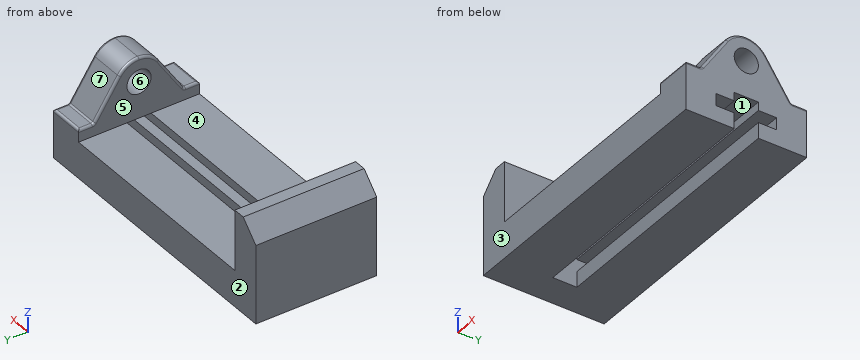
```python
from build123d import *

# Parameters (mm, degrees)
F0_W     = 127
F0_H     = 101.6
F1_DEPTH = 304.8
F2_W     = 234.95
F2_H     = 63.5
F3_DEPTH = 127.001
F4_R     = 12.7
F5_DEPTH = 273.05
F6_SIZE  = 19.05
F7_F1_R  = 2.54
F7_F2_R  = 2.54


with BuildPart() as f1:
    # F0 (on Right) → F1 (new body)
    with BuildSketch(Plane.YZ):
        with Locations((63.5, 50.8)):
            Rectangle(F0_W, F0_H)
    extrude(amount=-F1_DEPTH)

    # F2 (on face) → F3 (cut, through all)
    with BuildSketch(Plane.XZ):
        with Locations((-155.575, 69.85)):
            Rectangle(F2_W, F2_H)
    extrude(amount=-F3_DEPTH, mode=Mode.SUBTRACT)

    # F4 (on face) → F5 (cut, through all)
    with BuildSketch(Plane.YZ):
        with Locations((63.5, 76.2)):
            Circle(F4_R)
        Polygon((50.8, 16.51), (50.8, 0), (76.2, 0), (76.2, 16.51), (95.25, 16.51), (95.25, 29.21), (76.2, 29.21), (76.2, 38.1), (50.8, 38.1), (50.8, 29.21), (31.75, 29.21), (31.75, 16.51), align=None)
        with BuildLine():
            Line((0, 101.6), (0, 50.8))
            Line((0, 50.8), (15.875, 50.8))
            Line((15.875, 50.8), (42.4065743945, 90.3501730104))
            ThreePointArc((42.4065743945, 90.3501730104), (51.5470588235, 98.6117647059), (63.5, 101.6))
            Line((63.5, 101.6), (0, 101.6))
        make_face()
        with BuildLine():
            Line((127, 101.6), (63.5, 101.6))
            ThreePointArc((63.5, 101.6), (75.4529411765, 98.6117647059), (84.5934256055, 90.3501730104))
            Line((84.5934256055, 90.3501730104), (111.125, 50.8))
            Line((111.125, 50.8), (127, 50.8))
            Line((127, 50.8), (127, 101.6))
        make_face()
    extrude(amount=-F5_DEPTH, mode=Mode.SUBTRACT)

    # F6
    f6_edges = [f1.edges().sort_by_distance(p)[0] for p in [
        (-304.8, 63.5, 101.6),
    ]]
    chamfer(f6_edges, length=F6_SIZE)

    # F7: fillet of radius 2.54 on 6 edges, made by hand

    # F7_f1
    f7_f1_edges = [f1.edges().sort_by_distance(p)[0] for p in [
        (-19.05, 15.875, 50.8),
        (-19.05, 111.125, 50.8),
    ]]
    fillet(f7_f1_edges, radius=F7_F1_R)

    # F7_f2
    f7_f2_edges = [f1.edges().sort_by_distance(p)[0] for p in [
        (0, 29.5181251442, 71.1375778547),
        (-38.1, 29.5181251442, 71.1375778547),
        (-19.05, 127, 50.8),
        (-19.05, 0, 50.8),
        (-38.1, 63.5, 101.6),
        (-38.1, 97.4818748558, 71.1375778547),
        (0, 63.5, 101.6),
        (0, 97.4818748558, 71.1375778547),
        (0, 111.284372549, 51.0988235294),
        (-38.1, 111.284372549, 51.0988235294),
        (-38.1, 15.715627451, 51.0988235294),
        (0, 15.715627451, 51.0988235294),
    ]]
    fillet(f7_f2_edges, radius=F7_F2_R)


solid = f1.part
```
Could you check a few things on this model? Use its own coordinates, in mm. Face numbers are marked on the shaded views. A direction names the side the tool comes from. Give positions to 0.01 mm unless a question says otherwise; leave off trailing zeros. Loops run counter-clockwise (first coordinate to the right, second up) from the corner with the lowest first, then second, coordinate; pieces in that order, holes last. Notation, with made-up numbers: (72.25, 11.25) - (103.25, 11.25) arc R33 ccw to (103.25, 47.25) - close; hole circle Ø9 at (-4, 54.25). An arc over 180 degrees is marked (long way). Answer in a Markdown table with one row per item. Add a question column.
Q1. We'd pull the mould along Y, two halves only. Please class the marked faces 1, 2, 3 and 4: +Y half, -Y half, draft (parallel to the pull), parting line (faces both ways), or undercut.
Q2. Please list where these lines run through material, in increasing order: L1, parallel to Z at x = -14, y = 63.5; L2, parallel to Y at x = -145, z = 4; L3, parallel to Y at x = -151.5, z = 29. Write a range as from..to.
Q3. If we section it at B-B (y = 67.5): State how many separate pieces and enclosed holes the cut face has, plus the area to 3 significant figures.
Q4. For pin 1 (9.5 mm diameter, centred on x = -25, y = 11, fed in from +Z); pin 2 (12.5 mm diameter, centred on x = -11, y = 63, fed in from -Z); pin 3 (20.5 mm diameter, centred on y = 63.5, z = 76.2, fed in from +X), each with a flat end and sliding along its axis, tell me the tip position at first contact or that it passes through.
Q5. If we section it at A-A (x = -189): List the corners of the cut face in (y, z) for me, plus the area to 3 significant figures.
Q6. Which directions (+Z, -Z, +X, -X, +Y, -Y) give clear straight access to the entire face, cutting with the end or side of a thin tool? Please do the marked faces 5, 6 and 7.
The answers:
| question | item | result |
|---|---|---|
| 1 | face 1 | undercut |
| 1 | face 2 | +Y half |
| 1 | face 3 | -Y half |
| 1 | face 4 | draft |
| 2 | L1 | z = 38.1..63.5, 88.9..101.6 |
| 2 | L2 | y = 0..50.8, 76.2..127 |
| 2 | L3 | y = 0..31.75, 95.25..127 |
| 3 | separate pieces | 3 |
| 3 | enclosed holes | 0 |
| 3 | area | 4,530 mm^2 |
| 4 | pin 1 | stops at z = 51.12 |
| 4 | pin 2 | stops at z = 38.1 |
| 4 | pin 3 | stops at x = -273.05 |
| 5 | outline | (0, 0) - (50.8, 0) - (50.8, 16.51) - (31.75, 16.51) - (31.75, 29.21) - (50.8, 29.21) - (50.8, 38.1) - (0, 38.1) - close; (76.2, 0) - (127, 0) - (127, 38.1) - (76.2, 38.1) - (76.2, 29.21) - (95.25, 29.21) - (95.25, 16.51) - (76.2, 16.51) - close |
| 5 | area | 3,390 mm^2 |
| 6 | face 5 | +Z, +Y, -Y |
| 6 | face 6 | +X |
| 6 | face 7 | +Z, +X, +Y |
